from build123d import *

# Parameters (mm, degrees)
F1_DEPTH  = 18
F2_W      = 4
F2_H      = 5
F3_DEPTH  = 2
F2_R      = 2.25
F4_DEPTH  = 25
F5_R      = 4.5
F6_DEPTH  = 25
F7_R      = 2.25
F8_DEPTH  = 25
F7_W      = 4
F7_H      = 5
F9_DEPTH  = 2
F10_R     = 4.5
F11_DEPTH = 25


with BuildPart() as f1:
    # F0 (on Top) → F1 (new body)
    with BuildSketch(Plane.XY):
        Polygon((0, 38), (0, 0), (38, 0), (38, 5), (10, 5), (5, 10), (5, 38), align=None)
    extrude(amount=F1_DEPTH)

    # F2 (on face) → F3 (join)
    with BuildSketch(Plane.XZ):
        with Locations((2, 9)):
            Rectangle(F2_W, F2_H)
        with Locations((36, 9)):
            Rectangle(F2_W, F2_H)
    extrude(amount=F3_DEPTH)

    # F2 (on face) → F4 (cut)
    with BuildSketch(Plane.XZ):
        with Locations((14, 9)):
            Circle(F2_R)
        with Locations((26, 9)):
            Circle(F2_R)
    extrude(amount=-F4_DEPTH, mode=Mode.SUBTRACT)

    # F5 (on face) → F6 (cut)
    with BuildSketch(Plane(origin=(0, 5, 0), x_dir=(-1, 0, 0), z_dir=(0, 1, 0))):
        with Locations((-14, 9)):
            Circle(F5_R)
    extrude(amount=F6_DEPTH, mode=Mode.SUBTRACT)

    # F7 (on face) → F8 (cut)
    with BuildSketch(Plane(origin=(0, 0, 0), x_dir=(0, -1, 0), z_dir=(-1, 0, 0))):
        with Locations((-14, 9)):
            Circle(F7_R)
        with Locations((-26, 9)):
            Circle(F7_R)
    extrude(amount=-F8_DEPTH, mode=Mode.SUBTRACT)

    # F7 (on face) → F9 (join)
    with BuildSketch(Plane(origin=(0, 0, 0), x_dir=(0, -1, 0), z_dir=(-1, 0, 0))):
        Polygon((2, 6.5), (2, 11.5), (0, 11.5), (-4, 11.5), (-4, 6.5), (0, 6.5), align=None)
        with Locations((-36, 9)):
            Rectangle(F7_W, F7_H)
    extrude(amount=F9_DEPTH)

    # F10 (on face) → F11 (cut)
    with BuildSketch(Plane.YZ.offset(5)):
        with Locations((14, 9)):
            Circle(F10_R)
    extrude(amount=F11_DEPTH, mode=Mode.SUBTRACT)


solid = f1.part
Build history of the part. All positions in model axes, mm. A direction names the side the tool comes from. Coordinates: 2 decimals unless noted, no trailing zeros. Write each loop counter-clockwise with the first axis right and the second up, starting at its lowest first coordinate (ties: lowest second). Pieces come first, ordered by that corner, then holes. Notation, with made-up numbers: (64, -2) -> (112, -2) arc R24 ccw to (112, 29) -> close; hole circle Ø6 at (46, 43). An arc over 180 degrees is marked (long way). Use CSV: the item, a comma, the result in double quotes. Start each with the question number.
Q1. Flat gauge pins, fed straight in: pin 1 Ø7 at (x, z) = (14, 9) entering from -Y; pin 2 Ø1.5 at (x, y) = (25, 7.5) entering from -Z; pin 3 Ø0.6 at (x, y) = (-1.5, 36) entering from -Z; pin 4 Ø5.5 at (y, z) = (24, 10) entering from -X. Where does each tip first touch, or does it go through?
Q2. Cut at A-A, the plane x = 26. List the corners of the cut face in (y, z).
Q3. Drill centre lines: probe 1 along Z at (x, y) = (2.1, 26); probe 2 along Y at (x, z) = (32.5, 3.5); probe 3 along X at (y, z) = (0.5, 4.25). Where is each one in solid material? Low to high.
Q4. Cut at D-D, the plane x = 35. List the corners of the cut face in (y, z).
Q5. Pull direction Z, two halves, no side cores. Call faces 4 (the cylindrical face through (27.21, 2.465, 10.897)), 5 (the flat face through (36, -2, 9)), 6 (the flat face through (4.8, 12.1, 18)): released by +Z, released by -Z, zero draft, split by the parting line, or undercut.
Q6. 3-axis set-ups, long thin cutter, end or side, ignore diameter. For faces 1 (the flat face through (-1, 34, 9)), 2 (the flat face through (-1, 36, 6.5)), 3 (the flat face through (36, -1, 11.5)): which of +Z, -Z, +X, -X, +Y, -Y reach the whole face in a straight line?
Q7. Cut at C-C, the plane z = 14.25. List the corners of the cut face in (x, y).
Checked values:
1,pin 1,"stops at y = 0"
1,pin 2,"passes through"
1,pin 3,"stops at z = 6.5"
1,pin 4,"stops at x = 0"
2,outline,"(0, 0) -> (5, 0) -> (5, 6.75) -> (0, 6.75) -> close; (0, 11.25) -> (5, 11.25) -> (5, 18) -> (0, 18) -> close"
3,probe 1,"z = 0 to 6.75, 11.25 to 18"
3,probe 2,"y = 0 to 5"
3,probe 3,"x = 0 to 38"
4,outline,"(-2, 6.5) -> (0, 6.5) -> (0, 0) -> (5, 0) -> (5, 18) -> (0, 18) -> (0, 11.5) -> (-2, 11.5) -> close"
5,face 4,"undercut"
5,face 5,"zero draft"
5,face 6,"released by +Z"
6,face 1,"+Z, -Z, -X"
6,face 2,"-Z, -X, +Y, -Y"
6,face 3,"+Z, +X, -X, -Y"
7,outline,"(0, 0) -> (38, 0) -> (38, 5) -> (10, 5) -> (5, 10) -> (5, 38) -> (0, 38) -> close"
